Input: part model. Units: mm. Frame: model coordinates. A direction names the side the tool comes from. Give positions to 0.01 mm unless a question says otherwise; leave off trailing zeros. Loops run counter-clockwise (first coordinate to the right, second up) from the corner with the lowest first, then second, coordinate; pieces in that order, holes last. Notation, with made-up numbers: M 72.5,72.25 L 112.5,72.25 A24 cw 112.5,86.25 Z; hole C 86.5,62.25 d6. An arc over 180 degrees is marked long. Answer as a JSON object with one key per item and string values. Group by question number.
1) Access query for faces 1 (the flat face through (1.2, 1.2, 7)), 2 (the flat face through (2, 0, 1)), 3 (the conical face through (0.06, 2.82, 0.12)), 4 (the conical face through (0.02, -1.35, 0.18)). Directions: +Z, -Z, +X, -X, +Y, -Y. A direction counts if a zero-diameter tool reaches every point of the face in a straight line with its end or side. Return the directions, or none.
2) First-contact query: P1, Ø0.5, axis at x = -2.5, z = 0.5, coming from the -Y side; P2, Ø0.5, axis at x = 2, z = 0.5, coming from the -Y side; P3, Ø1, axis at x = -1.5, z = 11, coming from the -Y side. Flat tips, straight axial feed; report the tip coordinate or a pass-through.
3) Draft query along X for faces 5 (the flat face through (-2, 0, 1)), 6 (the cylindrical face through (-1.5, 0.07, 9.89)), 7 (the cylindrical face through (-0.369, 1.173, 3.19)). Return one class per face: +X half, -X half, draft (parallel to the pull), parting line (faces both ways), or undercut.
4) Section query B-B on y = 0. Return loops of the section in (x, z), plus the area to 3 significant figures.
5) Section query D-D on z = 9.25. Return loops of the section in (x, y).
6) Section query C-C on z = 4.25. Return loops of the section in (x, y).
7) Section query A-A on x = 0. Return loops of the section in (y, z).
8) Ray query, L1, parallel to Y at x = 0, z = 2.1; L2, parallel to Z at x = -0.7, y = -0.75. Return the intervals inside material, ascending.
Autodesk Inventor part; units mm, degrees
ref_plane "YZ Plane" through (0, 0, 0) normal (1, 0, 0) x (0, 1, 0)
ref_plane "XZ Plane" through (0, 0, 0) normal (0, 1, 0) x (-1, 0, 0)
ref_plane "XY Plane" through (0, 0, 0) normal (0, 0, 1) x (1, 0, 0)
sketch "Sketch1" plane through (0, 0, 0) normal (0, 1, 0) x (-1, 0, 0)
  line L0 (0, 0) -> (-3, 0)
  line L1 (-3, 0) -> (-3, 7)
  line L2 (-3, 7) -> (-1.5, 7)
  line L3 (-1.5, 7) -> (-1.5, 13)
  line L4 (-1.5, 13) -> (0, 13)
  line L5 (0, 13) -> (0, 0)
  dimension "d1" = 6
  dimension "d2" = 7
  dimension "d3" = 3
  dimension "d4" = 6
revolve "Revolution1" add sketch "Sketch1" angle 360 about axis through (0, 0, 13) along (0, 0, -1)
sketch "Sketch2" plane through (0, 0, 0) normal (0, 0, -1) x (-1, 0, 0)
  line L0 (-3, -0.5) -> (3, -0.5)
  line L1 (3, -0.5) -> (3, 0.5)
  line L2 (3, 0.5) -> (-3, 0.5)
  line L3 (-3, 0.5) -> (-3, -0.5)
  line L4 (-3, -0.5) -> (3, 0.5) construction
  line L5 (3, -0.5) -> (-3, 0.5) construction
  circle A0 centre (0, 0) radius 3
  dimension "d6" = 1
extrude "Extrusion1" cut sketch "Sketch2" against normal blind 1 contours L3 A0 L0 | A0 L2 L0 | L3 L2 A0 | A0 L1 L0 | A0 L2 L1
hole "Hole1" at (0, 0, 0) direction (0, 0, 1) diameter 2.459 depth 6
thread "Thread1"
chamfer "Chamfer1" distance 0.3 angle 45 7 edges at (-3, 0, 7) (0, 3, 0) (0, -3, 0) (0, -1.2295, 0) (-0.6697, 1.0311, 0) (0.6697, 1.0311, 0) (-1.5, 0, 13)
properties part number "BRU-307S" material "Stainless Steel AISI 304"
Output:
{
 "1": {"face 1": "+Z", "face 2": "-Z, +X, -X", "face 3": "-Z, +Y", "face 4": "-Z"},
 "2": {"P1": "stops at y = -1.98", "P2": "stops at y = -2.44", "P3": "stops at y = -1.12"},
 "3": {"face 5": "draft", "face 6": "parting line", "face 7": "undercut"},
 "4": {"outline": "M -3,1 L -1.23,1 L -1.23,6 L 1.23,6 L 1.23,1 L 3,1 L 3,6.7 L 2.7,7 L 1.5,7 L 1.5,12.7 L 1.2,13 L -1.2,13 L -1.5,12.7 L -1.5,7 L -2.7,7 L -3,6.7 Z", "area": "41.5 mm^2"},
 "5": {"outline": "C 0,0 d3"},
 "6": {"outline": "C 0,0 d6; hole C 0,0 d2.46"},
 "7": {"outline": "M -3,0.3 L -2.7,0 L -1.53,0 L -1.23,0.3 L -1.23,6 L 1.23,6 L 1.23,0.3 L 1.53,0 L 2.7,0 L 3,0.3 L 3,6.7 L 2.7,7 L 1.5,7 L 1.5,12.7 L 1.2,13 L -1.2,13 L -1.5,12.7 L -1.5,7 L -2.7,7 L -3,6.7 Z"},
 "8": {"L1": "y = -3 to -1.23, 1.23 to 3", "L2": "z = 6 to 13"}
}
